Input: part model. Units: mm. Frame: model coordinates. A direction names the side the tool comes from. Coordinates: 2 decimals unless noted, no trailing zeros. Write each loop counter-clockwise with the first axis right and the second up, starting at its lowest first coordinate (ties: lowest second). Pieces come first, ordered by that corner, then holes. Notation, with made-up numbers: (71, 23.25) - (121, 23.25) arc R19 cw to (121, 50.25) - close; hole circle Ø3 at (-22, -28). An arc over 180 degrees is marked (long way). Use a Markdown table: item, result. Add a question column.
Q1. Material intervals for probe 1 along X at (y, z) = (-197.5, -88); probe 2 along Z at (x, y) = (1335, -170); probe 3 along Z at (x, y) = (1073.5, 3), sorted ascending. Write a range as from..to.
Q2. Set-up query: faces 5 (the face through (1177.5, -22.6, 101.9)), 6 (the face through (1000, 108, 4)). Return all of +Z, -Z, +X, -X, +Y, -Y with unobstructed straight access to the full face (end or side cutting, diameter ignored); none if empty.
Q3. Section query D-D (z = -213.5). Return the cut outline in (x, y).
Q4. Section query A-A (y = 0). Return the cut outline in (x, z), then the cut area to 3 significant figures.
Q5. Section query C-C (x = 1261). Return the cut outline in (y, z), then the cut area to 3 significant figures.
Q6. Pin query (flat end, axial travel): P1, Ø12, axis at y = 128, z = -92, coming from the +X side; P2, Ø6, axis at x = 1016, y = 23, coming from the +Z side. Return the tip coordinate at first contact, or that it passes through.
Q7. Mould query, pull axis X, two halves, no side actions, for faces 1 (the face through (493, 250, 4)), 2 (the face through (1040, -1, -1)), 3 (the face through (0, -3, 4)), 4 (the face through (1158.356, 133.143, -41.929)). Classes: released by +X, released by -X, zero draft, split by the parting line, or undercut.
from build123d import *

# Parameters (mm, degrees)
SKETCH1_W                = 1000
SKETCH1_H                = 500
BOSS_EXTRUDE1_DEPTH      = 250
BOSS_EXTRUDE1_DEPTH_BACK = 250


with BuildPart() as part:
    # Sketch1 → Boss-Extrude1 (new body, two sides)
    with BuildSketch(Plane.XY) as boss_extrude1_sk:
        with Locations((500, 0)):
            Rectangle(SKETCH1_W, SKETCH1_H)
    extrude(amount=BOSS_EXTRUDE1_DEPTH)
    extrude(boss_extrude1_sk.sketch, amount=-BOSS_EXTRUDE1_DEPTH_BACK)

    # Sketch3 → Revolve1 (revolve)
    with BuildSketch(Plane.XY):
        Polygon((1000, 0), (1000, 100), (1400, 200), (1400, 160), (1040, 70), (1040, 0), align=None)
    revolve(axis=Axis((1040, 0, 0), (-1, 0, 0)))


solid = part.part
Values follow:
| question | item | result |
|---|---|---|
| 1 | probe 1 | 0..1000 |
| 1 | probe 2 | -69.74..69.74 |
| 1 | probe 3 | -118.34..-78.32, 78.32..118.34 |
| 2 | face 5 | +X |
| 2 | face 6 | none |
| 3 | outline | (0, -250) - (1000, -250) - (1000, 250) - (0, 250) - close |
| 4 | outline | (0, -250) - (1000, -250) - (1000, -100) - (1400, -200) - (1400, -160) - (1040, -70) - (1040, 70) - (1400, 160) - (1400, 200) - (1000, 100) - (1000, 250) - (0, 250) - close |
| 4 | area | 537,000 mm2 |
| 5 | outline | circle Ø330.5 at (0, 0); hole circle Ø250.5 at (0, 0) |
| 5 | area | 36,500 mm2 |
| 6 | P1 | x = 1400 |
| 6 | P2 | z = 102.43 |
| 7 | face 1 | zero draft |
| 7 | face 2 | released by +X |
| 7 | face 3 | released by -X |
| 7 | face 4 | undercut |
